Could you check a few things on this model? Use its own coordinates, in mm. Face numbers are marked on the shaded views. Coordinates: 2 decimals unless noted, no trailing zeros. Order: outer loops, then holes, each group sorted by start corner. A loop starts at its lowest first (then second) coordinate and runs counter-clockwise, first axis right, second up. Notation, with made-up numbers: (11.5, 1) - (31.5, 1) arc R5 cw to (31.5, 8) - close; hole circle Ø9 at (34, -12.75). An arc over 180 degrees is marked (long way). One line per item, written item: value.
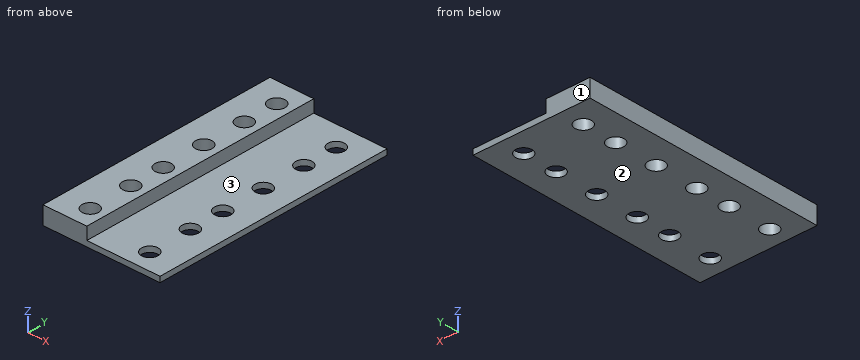
from build123d import *

# Parameters (mm, degrees)
SKETCH1_W           = 42.75
SKETCH1_H           = 88.9
SKETCH1_W_2         = 9.5
SKETCH1_H_2         = 9.5
BOSS_EXTRUDE1_DEPTH = 2
SKETCH2_W           = 9.5
SKETCH2_H           = 9.5
SKETCH2_R           = 3
BOSS_EXTRUDE2_DEPTH = 2
SKETCH3_W           = 16
SKETCH3_H           = 88.9
SKETCH3_R           = 3
BOSS_EXTRUDE3_DEPTH = 6.5


with BuildPart() as part:
    # Sketch1 → Boss-Extrude1 (new body)
    with BuildSketch(Plane.XY):
        with Locations((-3.875, 44.45)):
            Rectangle(SKETCH1_W, SKETCH1_H)
        with Locations((7, 67.59)):
            Rectangle(SKETCH1_W_2, SKETCH1_H_2, mode=Mode.SUBTRACT)
        with Locations((7, 80.29)):
            Rectangle(SKETCH1_W_2, SKETCH1_H_2, mode=Mode.SUBTRACT)
        with Locations((-14.75, 80.29)):
            Rectangle(SKETCH1_W_2, SKETCH1_H_2, mode=Mode.SUBTRACT)
        with Locations((-14.75, 67.59)):
            Rectangle(SKETCH1_W_2, SKETCH1_H_2, mode=Mode.SUBTRACT)
        with Locations((-14.75, 7.25)):
            Rectangle(SKETCH1_W_2, SKETCH1_H_2, mode=Mode.SUBTRACT)
        with Locations((7, 51.71)):
            Rectangle(SKETCH1_W_2, SKETCH1_H_2, mode=Mode.SUBTRACT)
        with Locations((-14.75, 51.71)):
            Rectangle(SKETCH1_W_2, SKETCH1_H_2, mode=Mode.SUBTRACT)
        with Locations((7, 7.25)):
            Rectangle(SKETCH1_W_2, SKETCH1_H_2, mode=Mode.SUBTRACT)
        with Locations((7, 23.13)):
            Rectangle(SKETCH1_W_2, SKETCH1_H_2, mode=Mode.SUBTRACT)
        with Locations((-14.75, 23.13)):
            Rectangle(SKETCH1_W_2, SKETCH1_H_2, mode=Mode.SUBTRACT)
        with Locations((7, 35.83)):
            Rectangle(SKETCH1_W_2, SKETCH1_H_2, mode=Mode.SUBTRACT)
        with Locations((-14.75, 35.83)):
            Rectangle(SKETCH1_W_2, SKETCH1_H_2, mode=Mode.SUBTRACT)
    extrude(amount=BOSS_EXTRUDE1_DEPTH)

    # Sketch2 → Boss-Extrude2 (add)
    with BuildSketch(Plane(origin=(0, 0, 0), x_dir=(-1, 0, 0), z_dir=(0, 0, -1))):
        with Locations((-7, 80.29)):
            Rectangle(SKETCH2_W, SKETCH2_H)
        with Locations((-7, 80.29)):
            Circle(SKETCH2_R, mode=Mode.SUBTRACT)
        with Locations((14.75, 80.29)):
            Rectangle(SKETCH2_W, SKETCH2_H)
        with Locations((14.75, 80.29)):
            Circle(SKETCH2_R, mode=Mode.SUBTRACT)
        with Locations((-7, 67.59)):
            Rectangle(SKETCH2_W, SKETCH2_H)
        with Locations((-7, 67.59)):
            Circle(SKETCH2_R, mode=Mode.SUBTRACT)
        with Locations((14.75, 67.59)):
            Rectangle(SKETCH2_W, SKETCH2_H)
        with Locations((14.75, 67.59)):
            Circle(SKETCH2_R, mode=Mode.SUBTRACT)
        with Locations((-7, 51.71)):
            Rectangle(SKETCH2_W, SKETCH2_H)
        with Locations((-7, 51.71)):
            Circle(SKETCH2_R, mode=Mode.SUBTRACT)
        with Locations((14.75, 51.71)):
            Rectangle(SKETCH2_W, SKETCH2_H)
        with Locations((14.75, 51.71)):
            Circle(SKETCH2_R, mode=Mode.SUBTRACT)
        with Locations((-7, 35.83)):
            Rectangle(SKETCH2_W, SKETCH2_H)
        with Locations((-7, 35.83)):
            Circle(SKETCH2_R, mode=Mode.SUBTRACT)
        with Locations((14.75, 35.83)):
            Rectangle(SKETCH2_W, SKETCH2_H)
        with Locations((14.75, 35.83)):
            Circle(SKETCH2_R, mode=Mode.SUBTRACT)
        with Locations((-7, 23.13)):
            Rectangle(SKETCH2_W, SKETCH2_H)
        with Locations((-7, 23.13)):
            Circle(SKETCH2_R, mode=Mode.SUBTRACT)
        with Locations((14.75, 23.13)):
            Rectangle(SKETCH2_W, SKETCH2_H)
        with Locations((14.75, 23.13)):
            Circle(SKETCH2_R, mode=Mode.SUBTRACT)
        with Locations((14.75, 7.25)):
            Rectangle(SKETCH2_W, SKETCH2_H)
        with Locations((14.75, 7.25)):
            Circle(SKETCH2_R, mode=Mode.SUBTRACT)
        with Locations((-7, 7.25)):
            Rectangle(SKETCH2_W, SKETCH2_H)
        with Locations((-7, 7.25)):
            Circle(SKETCH2_R, mode=Mode.SUBTRACT)
    extrude(amount=-BOSS_EXTRUDE2_DEPTH)

    # Sketch3 → Boss-Extrude3 (add)
    with BuildSketch(Plane(origin=(0, 0, 0), x_dir=(-1, 0, 0), z_dir=(0, 0, -1))):
        with Locations((17.25, 44.45)):
            Rectangle(SKETCH3_W, SKETCH3_H)
        with Locations((14.75, 80.29)):
            Circle(SKETCH3_R, mode=Mode.SUBTRACT)
        with Locations((14.75, 67.59)):
            Circle(SKETCH3_R, mode=Mode.SUBTRACT)
        with Locations((14.75, 51.71)):
            Circle(SKETCH3_R, mode=Mode.SUBTRACT)
        with Locations((14.75, 35.83)):
            Circle(SKETCH3_R, mode=Mode.SUBTRACT)
        with Locations((14.75, 23.13)):
            Circle(SKETCH3_R, mode=Mode.SUBTRACT)
        with Locations((14.75, 7.25)):
            Circle(SKETCH3_R, mode=Mode.SUBTRACT)
    extrude(amount=-BOSS_EXTRUDE3_DEPTH)


solid = part.part
Item 1: I'm going to push flat-ended pins straight in: pin 1 Ø8 at (x, y) = (7, 80.29) entering from +Z; pin 2 Ø2 at (y, z) = (11.5, 4) entering from +X. Where does each tip first touch, or does it pass through?
Conclusion:
pin 1: z = 2
pin 2: x = -9.25
Item 2: If I drill on probe 1 along X at (y, z) = (35, 1.5); probe 2 along Z at (x, y) = (0.5, 24); probe 3 along X at (y, z) = (7, 2.5), over which ranges is the centre line in solid material (lowest first)?
Conclusion:
probe 1: -25.25 to -17.63, -11.87 to 4.12, 9.88 to 17.5
probe 2: 0 to 2
probe 3: -25.25 to -17.74, -11.76 to -9.25
Item 3: Thinking about a two-plate mould opening in Z: for the marked faces 1, 2 and 3, which applies, pulls with the +Z half, pulls with the -Z half, needs draft (parallel to the pull), parting line crosses it, or undercut?
Conclusion:
face 1: needs draft
face 2: pulls with the -Z half
face 3: pulls with the +Z half
Item 4: I want a section at B-B on z = 3.5. Please give me the cut outline in (x, y).
Conclusion:
outline: (-25.25, 0) - (-9.25, 0) - (-9.25, 88.9) - (-25.25, 88.9) - close; hole circle Ø6 at (-14.75, 7.25); hole circle Ø6 at (-14.75, 23.13); hole circle Ø6 at (-14.75, 35.83); hole circle Ø6 at (-14.75, 51.71); hole circle Ø6 at (-14.75, 67.59); hole circle Ø6 at (-14.75, 80.29)
Item 5: I want a section at C-C on x = 7. Please give me the cut outline in (y, z), then the cut area to 3 significant figures.
Conclusion:
outline: (0, 0) - (4.25, 0) - (4.25, 2) - (0, 2) - close; (10.25, 0) - (20.13, 0) - (20.13, 2) - (10.25, 2) - close; (26.13, 0) - (32.83, 0) - (32.83, 2) - (26.13, 2) - close; (38.83, 0) - (48.71, 0) - (48.71, 2) - (38.83, 2) - close; (54.71, 0) - (64.59, 0) - (64.59, 2) - (54.71, 2) - close; (70.59, 0) - (77.29, 0) - (77.29, 2) - (70.59, 2) - close; (83.29, 0) - (88.9, 0) - (88.9, 2) - (83.29, 2) - close
area: 106 mm²
Item 6: I want a section at A-A on y = 51.71. Please give me the cut outline in (x, z), then the cut area to 4 significant figures.
Conclusion:
outline: (-25.25, 0) - (-17.75, 0) - (-17.75, 6.5) - (-25.25, 6.5) - close; (-11.75, 0) - (4, 0) - (4, 2) - (-9.25, 2) - (-9.25, 6.5) - (-11.75, 6.5) - close; (10, 0) - (17.5, 0) - (17.5, 2) - (10, 2) - close
area: 106.5 mm²
Item 7: I want a section at D-D on y = 28.5. Please give me the cut outline in (x, z), then the cut area to 4 significant figures.
Conclusion:
outline: (-25.25, 0) - (17.5, 0) - (17.5, 2) - (-9.25, 2) - (-9.25, 6.5) - (-25.25, 6.5) - close
area: 157.5 mm²
